Design review of the part built by this model. Coordinates are the model's own, in mm. Coordinates: 2 decimals unless noted, no trailing zeros. Loops run counter-clockwise (first coordinate to the right, second up) from the corner with the lowest first, then second, coordinate; pieces in that order, holes last. Notation, with made-up numbers: (-8.5, -40) - (8.5, -40) arc R12 ccw to (8.5, -18) - close; hole circle Ø4 at (88.25, 1). An arc over 180 degrees is marked (long way). Answer in a Markdown table with one row per item. Add a question column.
(1) Clearance check with a flat-ended pin moving along its axis: pin 1 (3.5 mm diameter, centred on x = 7.66, z = 4.42, fed in from +Y). State where the tip first meets the part, or that it passes through.
(2) We need section A-A, the plane z = -16.85. Write out the cut boundary in (x, y).
(3) We need section B-B, the plane y = 0.9. Give the number of separate pieces and of enclosed holes in the cut face, plus the area to 3 significant figures.
(4) To check wall thickness, follow L1, parallel to Z at x = 0, y = 0.6; L2, parallel to X at y = 0.45, z = 4; L3, parallel to Z at x = 23.5, y = 1.1. State the ranges of each line that lie inside material, in increasing order. Write a range as [from, to].
from build123d import *

# Parameters (mm, degrees)
SKETCH1_R           = 26
BOSS_EXTRUDE1_DEPTH = 2
SKETCH2_R           = 3.25
SKETCH2_R_2         = 1.9
CUT_EXTRUDE1_DEPTH  = 3
CUT_EXTRUDE2_DEPTH  = 10
CIRPATTERN1_COUNT   = 20


with BuildPart() as part:
    # Sketch1 → Boss-Extrude1 (new body)
    with BuildSketch(Plane(origin=(0, 0, 0), x_dir=(1, 0, 0), z_dir=(0, 1, 0))):
        Circle(SKETCH1_R)
    extrude(amount=BOSS_EXTRUDE1_DEPTH)

    # Sketch2 → Cut-Extrude1 (cut, through all)
    with BuildSketch(Plane(origin=(0, 2, 0), x_dir=(1, 0, 0), z_dir=(0, 1, 0))):
        Circle(SKETCH2_R)
        with Locations((0, 8.85)):
            Circle(SKETCH2_R_2)
        with Locations((7.664324823, -4.425)):
            Circle(SKETCH2_R_2)
        with Locations((-7.664324823, -4.425)):
            Circle(SKETCH2_R_2)
        with Locations((0, 16.85)):
            Circle(SKETCH2_R_2)
    extrude(amount=-CUT_EXTRUDE1_DEPTH, mode=Mode.SUBTRACT)

    # Sketch5 → Cut-Extrude2 (cut)
    with BuildSketch(Plane(origin=(0, 2, 0), x_dir=(1, 0, 0), z_dir=(0, 1, 0))):
        with BuildLine():
            ThreePointArc((-7.591229417, 24.867111532), (-7.001593879, 24.012811344), (-6.503694096, 23.101990458))
            Line((-6.503694096, 23.101990458), (-6.252916986, 22.580637882))
            ThreePointArc((-6.252916986, 22.580637882), (-3.583333333, 21.199285889), (-1.516070361, 23.381311098))
            Line((-1.516070361, 23.381311098), (-1.450578836, 23.95612283))
            ThreePointArc((-1.450578836, 23.95612283), (-1.279700655, 24.979987824), (-1.003606428, 25.980623051))
            ThreePointArc((-1.003606428, 25.980623051), (-4.333333333, 25.636345727), (-7.591229417, 24.867111532))
        make_face()
    cut_extrude2 = extrude(amount=-CUT_EXTRUDE2_DEPTH, mode=Mode.SUBTRACT)

    # CirPattern1: Cut-Extrude2 ×20 about axis
    cirpattern1_axis = Axis((0, 0, 0), (0, 1, 0))
    for i in range(1, CIRPATTERN1_COUNT):
        add(cut_extrude2.rotate(cirpattern1_axis, i * 360 / CIRPATTERN1_COUNT), mode=Mode.SUBTRACT)


solid = part.part
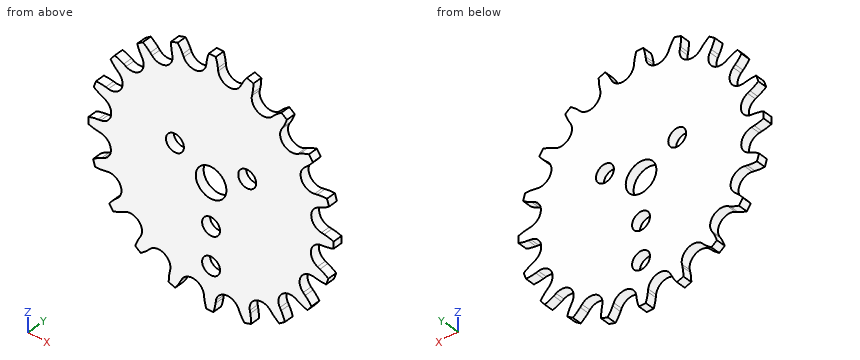
Responses:
| question | item | result |
|---|---|---|
| 1 | pin 1 | passes through |
| 2 | outline | (-14.65, 0) - (-1.9, 0) - (-1.9, 2) - (-14.65, 2) - close; (1.9, 0) - (14.31, 0) - (14.31, 2) - (1.9, 2) - close |
| 3 | separate pieces | 1 |
| 3 | enclosed holes | 5 |
| 3 | area | 1,620 mm2 |
| 4 | L1 | z = [-26, -18.75], [-14.95, -10.75], [-6.95, -3.25], [3.25, 26] |
| 4 | L2 | x = [-21.16, -9.52], [-5.81, 5.81], [9.52, 21.29] |
| 4 | L3 | z = [-8.95, -6.71], [-1.5, 1.02], [6.15, 8.45] |
